Can you work these out from the model? Positions are in its coordinate system, mm. A direction names the side the tool comes from. Round coordinates to 2 decimals unless told otherwise and drop trailing zeros. Write each loop counter-clockwise with the first axis right and the second up, starting at its lowest first coordinate (ties: lowest second). Pieces come first, ordered by that corner, then holes. Notation, with made-up numbers: (56, 87) -> (70, 87) arc R24 cw to (70, 103) -> close; hole circle Ø4 at (19.5, -17.5). An arc over 180 degrees is marked (long way). Use CSV: the item, a comma, the result in double quotes.
```python
from build123d import *

# Parameters (mm, degrees)
BOSS_EXTRUDE1_DEPTH = 57
BOSS_EXTRUDE2_DEPTH = 14.3
CUT_EXTRUDE1_DEPTH  = 10


with BuildPart() as part:
    # Sketch1 → Boss-Extrude1 (new body)
    with BuildSketch(Plane.XY):
        Polygon((0, 0), (-7.54, -7.54), (-38.5, -7.54), (-38.5, -2.54), (-9.611067812, -2.54), (0, 7.071067812), (9.611067812, -2.54), (38.5, -2.54), (38.5, -7.54), (7.54, -7.54), align=None)
    extrude(amount=BOSS_EXTRUDE1_DEPTH)

    # Sketch2 → Boss-Extrude2 (add)
    with BuildSketch(Plane.XY.offset(57)):
        Polygon((-7.54, -7.54), (0, 0), (7.54, -7.54), align=None)
    extrude(amount=-BOSS_EXTRUDE2_DEPTH)

    # Sketch3 → Cut-Extrude1 (cut)
    with BuildSketch(Plane(origin=(0, -2.54, 0), x_dir=(1, 0, 0), z_dir=(0, 1, 0))):
        with BuildLine():
            Line((-28.500315349, -48.5), (-28.500315349, -54.5))
            ThreePointArc((-28.500315349, -54.5), (-27, -56.000315349), (-25.499684651, -54.5))
            Line((-25.499684651, -54.5), (-25.499684651, -48.5))
            ThreePointArc((-25.499684651, -48.5), (-27, -46.999684651), (-28.500315349, -48.5))
        make_face()
        with BuildLine():
            Line((25.499684651, -2.5), (25.499684651, -8.5))
            ThreePointArc((25.499684651, -8.5), (27, -10.000315349), (28.500315349, -8.5))
            Line((28.500315349, -8.5), (28.500315349, -2.5))
            ThreePointArc((28.500315349, -2.5), (27, -0.999684651), (25.499684651, -2.5))
        make_face()
        with BuildLine():
            Line((-28.500315349, -2.5), (-28.500315349, -8.5))
            ThreePointArc((-28.500315349, -8.5), (-27, -10.000315349), (-25.499684651, -8.5))
            Line((-25.499684651, -8.5), (-25.499684651, -2.5))
            ThreePointArc((-25.499684651, -2.5), (-27, -0.999684651), (-28.500315349, -2.5))
        make_face()
        with BuildLine():
            Line((25.499684651, -48.5), (25.499684651, -54.5))
            ThreePointArc((25.499684651, -54.5), (27, -56.000315349), (28.500315349, -54.5))
            Line((28.500315349, -54.5), (28.500315349, -48.5))
            ThreePointArc((28.500315349, -48.5), (27, -46.999684651), (25.499684651, -48.5))
        make_face()
    extrude(amount=-CUT_EXTRUDE1_DEPTH, mode=Mode.SUBTRACT)


solid = part.part
```
Q1. Please list where these lines run through material, in increasing order: probe 1 along X at (y, z) = (-3.75, 54.5); probe 2 along Y at (x, z) = (20.5, 5.5); probe 3 along X at (y, z) = (-4.75, 48).
Resolved:
probe 1,"x = -38.5 to -28.5, -25.5 to 25.5, 28.5 to 38.5"
probe 2,"y = -7.54 to -2.54"
probe 3,"x = -38.5 to -28.41, -25.59 to 25.59, 28.41 to 38.5"
Q2. On a 3-axis mill with a long thin cutter (end or side, diameter ignored), from which of +Z, -Z, +X, -X, +Y, -Y can I reach the whole of each face in a straight line? I mean faces 5 (the face through (-24, -2.54, 28)), 6 (the face through (27, -5, 56)), 7 (the face through (24, -2.54, 28)). Say none if no direction works.
Resolved:
face 5,"+Z, -Z, -X, +Y"
face 6,"+Y, -Y"
face 7,"+Z, -Z, +X, +Y"
Q3. Will these pins go through, and if not, where does the flat tip stop? P1, Ø3, axis at x = -25, z = 31, coming from the +Y side; P2, Ø4, axis at y = 3, z = 50, coming from the +X side; P3, Ø1.5, axis at y = 3.5, z = 16, coming from the -X side.
Resolved:
P1,"stops at y = -2.54"
P2,"stops at x = 6.07"
P3,"stops at x = -4.32"
Q4. Suppose I cut it at D-D (y = -1). Write out the boundary of the cut face in (x, z), and give its area (3 significant figures).
Resolved:
outline,"(-8.07, 0) -> (-1, 0) -> (-1, 42.7) -> (1, 42.7) -> (1, 0) -> (8.07, 0) -> (8.07, 57) -> (-8.07, 57) -> close"
area,"835 mm^2"
Q5. If we mould it in two halves opening along X, with no side actions, what happens to faces 1 (the face through (-4.87, 2.2, 28.1)), 2 (the face through (25.5, -5, 51)), 3 (the face through (-8, -7.54, 29)), 4 (the face through (0, -5, 42.7))? For each: released by +X, released by -X, zero draft, split by the parting line, or undercut.
Resolved:
face 1,"released by -X"
face 2,"undercut"
face 3,"zero draft"
face 4,"undercut"
Q6. Suppose I cut it at A-A (y = -5.75). Write out the boundary of the cut face in (x, z), and give its area (3 significant figures).
Resolved:
outline,"(-38.5, 0) -> (-5.75, 0) -> (-5.75, 42.7) -> (5.75, 42.7) -> (5.75, 0) -> (38.5, 0) -> (38.5, 57) -> (-38.5, 57) -> close; hole (-28.5, 2.5) arc R1.5 ccw to (-25.5, 2.5) -> (-25.5, 8.5) arc R1.5 ccw to (-28.5, 8.5) -> close; hole (-28.5, 48.5) arc R1.5 ccw to (-25.5, 48.5) -> (-25.5, 54.5) arc R1.5 ccw to (-28.5, 54.5) -> close; hole (25.5, 2.5) arc R1.5 ccw to (28.5, 2.5) -> (28.5, 8.5) arc R1.5 ccw to (25.5, 8.5) -> close; hole (25.5, 48.5) arc R1.5 ccw to (28.5, 48.5) -> (28.5, 54.5) arc R1.5 ccw to (25.5, 54.5) -> close"
area,"3,800 mm^2"
Q7. Suppose I cut it at B-B (x = 27). Write out the boundary of the cut face in (y, z).
Resolved:
outline,"(-7.54, 0) -> (-2.54, 0) -> (-2.54, 1) -> (-7.54, 1) -> close; (-7.54, 10) -> (-2.54, 10) -> (-2.54, 47) -> (-7.54, 47) -> close; (-7.54, 56) -> (-2.54, 56) -> (-2.54, 57) -> (-7.54, 57) -> close"
Q8. Suppose I cut it at C-C (z = 30.5). Write out the boundary of the cut face in (x, y), and give its area (3 significant figures).
Resolved:
outline,"(-38.5, -7.54) -> (-7.54, -7.54) -> (0, 0) -> (7.54, -7.54) -> (38.5, -7.54) -> (38.5, -2.54) -> (9.61, -2.54) -> (0, 7.07) -> (-9.61, -2.54) -> (-38.5, -2.54) -> close"
area,"421 mm^2"
